Design review of the part shown in the three views and the two pictorial views. Dimensions are in mm from the part's minimum x, y and z. A direction names the side the tool comes from. Round coordinates to 2 decimals unless told otherwise and drop trailing zeros. Loops run counter-clockwise (first coordinate to the right, second up) from the corner with the lowest first, then second, coordinate; pieces in that order, holes last. Notation, with made-up numbers: M 64.5,75.5 L 70.5,75.5 A13 cw 70.5,99.5 Z; hole C 4,16 d11. An arc over 180 degrees is marked long. One line per question, with ' | ' between items. Start each with the question number.
1) For probe 1 along Z at (x, y) = (10, 10.25); probe 2 along X at (y, z) = (4.5, 1.45); probe 3 along Z at (x, y) = (10.5, 3), list the stretches that pass through material, from the lowest coordinate up. Write a range as from..to.
2) We need section A-A (y = 13.5). Give the boundary of the cut face in (x, z), and give its area (3 significant figures).
3) For the marked faces 1 and 2, list the 3-axis set-ups (+Z, -Z, +X, -X, +Y, -Y) from which the entire face can be reached by the end or side of a thin tool; tool diameter is ignored.
4) We need section B-B (z = 1.9). Give the boundary of the cut face in (x, y), and give its area (3 significant figures).
5) We need section C-C (x = 7). Give the boundary of the cut face in (y, z), and give its area (3 significant figures).
6) For pin 1 Ø1 at (x, y) = (4.5, 14.5) entering from +Z, flat-tipped, find the tip position at first contact; note if it passes through.
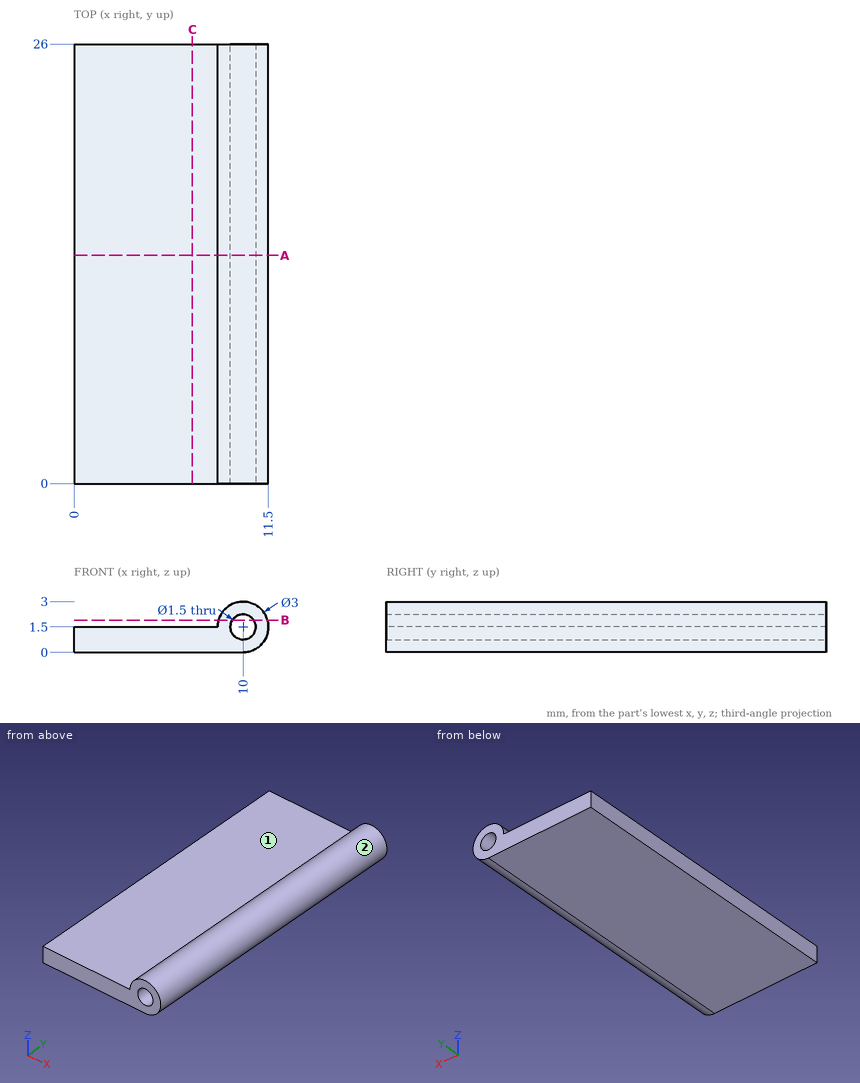
Answers below:
1) probe 1: 0..0.75, 2.25..3 | probe 2: 0..9.25, 10.75..11.5 | probe 3: 0.09..0.94, 2.06..2.91
2) outline: M 0,0 L 10,0 A1.5 ccw long 8.5,1.5 L 0,1.5 Z; hole C 10,1.5 d1.5 | area: 18.5 mm^2
3) face 1: +Z, -X, +Y, -Y | face 2: +Y, -Y
4) outline: M 8.55,0 L 9.37,0 L 9.37,26 L 8.55,26 Z; M 10.63,0 L 11.45,0 L 11.45,26 L 10.63,26 Z | area: 42.2 mm^2
5) outline: M 0,0 L 26,0 L 26,1.5 L 0,1.5 Z | area: 39.0 mm^2
6) pin 1: z = 1.5
